```python
from build123d import *

# Parameters (mm, degrees)
F0_W     = 139.7
F0_H     = 241.3
F0_R     = 7.14375
F1_DEPTH = 12.7
F3_W     = 101.6
F3_H     = 203.2
F4_DEPTH = 12.7
F5_W     = 139.7
F5_H     = 12.7
F6_DEPTH = 244.602
F9_DEPTH = 215.901


with BuildPart() as f1:
    # F0 (on Top) → F1 (new body)
    with BuildSketch(Plane.XY):
        Rectangle(F0_W, F0_H)
        with Locations((-50.8, -63.5)):
            Circle(F0_R, mode=Mode.SUBTRACT)
        with Locations((50.8, -63.5)):
            Circle(F0_R, mode=Mode.SUBTRACT)
        with Locations((-50.8, 63.5)):
            Circle(F0_R, mode=Mode.SUBTRACT)
        with Locations((50.8, 63.5)):
            Circle(F0_R, mode=Mode.SUBTRACT)
    extrude(amount=F1_DEPTH)


with BuildPart() as f4:
    # F3 (on offset) → F4 (new body)
    with BuildSketch(Plane.XY.offset(270.002)):
        with Locations((-19.05, 0)):
            Rectangle(F3_W, F3_H)
        with BuildLine():
            ThreePointArc((-57.15, -65.913), (-62.738, -60.325), (-57.15, -54.737))
            Line((-57.15, -54.737), (19.05, -54.737))
            ThreePointArc((19.05, -54.737), (24.638, -60.325), (19.05, -65.913))
            Line((19.05, -65.913), (-57.15, -65.913))
        make_face(mode=Mode.SUBTRACT)
        with BuildLine():
            Line((19.05, 54.737), (-57.15, 54.737))
            ThreePointArc((-57.15, 54.737), (-62.738, 60.325), (-57.15, 65.913))
            Line((-57.15, 65.913), (19.05, 65.913))
            ThreePointArc((19.05, 65.913), (24.638, 60.325), (19.05, 54.737))
        make_face(mode=Mode.SUBTRACT)
    extrude(amount=-F4_DEPTH)


with BuildPart() as f6:
    # F5 (on face) → F6 (new body, through all)
    with BuildSketch(Plane.XY.offset(12.7)):
        with Locations((0, 88.9)):
            Rectangle(F5_W, F5_H)
    extrude(amount=F6_DEPTH)


with BuildPart() as f6b:
    # F5 (on face) → F6, piece 2 (new body, through all)
    with BuildSketch(Plane.XY.offset(12.7)):
        with Locations((0, -88.9)):
            Rectangle(F5_W, F5_H)
    extrude(amount=F6_DEPTH)


with BuildPart() as f1_1:
    add(f1.part)

    # F7: union F6b, F6, F4
    add(f6b.part)
    add(f6.part)
    add(f4.part)

    # F8 (on face) → F9 (cut, through all)
    with BuildSketch(Plane.XZ.offset(95.25)):
        Polygon((69.85, 257.302), (31.75, 257.302), (69.85, 12.7), align=None)
    extrude(amount=-F9_DEPTH, mode=Mode.SUBTRACT)


solid = f1_1.part
```
For this review, take the finished solid that the model builds, in its own axes (mm). A direction names the side the tool comes from. Round coordinates to 2 decimals unless told otherwise and drop trailing zeros. Write each loop counter-clockwise with the first axis right and the second up, starting at its lowest first coordinate (ties: lowest second). Pieces come first, ordered by that corner, then holes. Notation, with made-up numbers: (55.5, 21) - (59.5, 21) arc R34 ccw to (59.5, 57) - close; hole circle Ø7 at (73.5, 87.25). An arc over 180 degrees is marked (long way). Use CSV: the item, a comma, the result in double quotes.
1) For faces 4 (the flat face through (31.75, -1, 264)), 5 (the flat face through (-17, 82.55, 133)), 6 (the flat face through (-20, -54.737, 264)), list the 3-axis set-ups (+Z, -Z, +X, -X, +Y, -Y) from which the entire face can be reached by the end or side of a thin tool; tool diameter is ignored.
Conclusion:
face 4,"+Z, +X, +Y, -Y"
face 5,"+X, -X"
face 6,"+Z"
2) Add section D-D on x = -24.5. Write out the cut boundary in (y, z).
Conclusion:
outline,"(-120.65, 0) - (120.65, 0) - (120.65, 12.7) - (95.25, 12.7) - (95.25, 257.3) - (101.6, 257.3) - (101.6, 270) - (65.91, 270) - (65.91, 257.3) - (82.55, 257.3) - (82.55, 12.7) - (-82.55, 12.7) - (-82.55, 257.3) - (-65.91, 257.3) - (-65.91, 270) - (-101.6, 270) - (-101.6, 257.3) - (-95.25, 257.3) - (-95.25, 12.7) - (-120.65, 12.7) - close; (-54.74, 257.3) - (54.74, 257.3) - (54.74, 270) - (-54.74, 270) - close"
3) Add section B-B on x = -50.8. Count the separate pieces of the cut face and the enclosed holes in it, and give its area (3 significant figures).
Conclusion:
separate pieces,"4"
enclosed holes,"0"
area,"11,200 mm^2"
4) The part is to be moulded in two halves that separate along X. For faces 1 (the flat face through (69.85, -2, 6)), 2 (the flat face through (-17, 95.25, 133)), 3 (the flat face through (-19, -65.913, 264)), say which applies: pulls with the +X half, pulls with the -X half, needs draft (parallel to the pull), parting line crosses it, or undercut.
Conclusion:
face 1,"pulls with the +X half"
face 2,"needs draft"
face 3,"undercut"
5) Add section A-A on y = -38. Write out the cut boundary in (x, z).
Conclusion:
outline,"(-69.85, 0) - (69.85, 0) - (69.85, 12.7) - (-69.85, 12.7) - close; (-69.85, 257.3) - (31.75, 257.3) - (31.75, 270) - (-69.85, 270) - close"
6) Wall thickness on line 1 along Y through (x, z) = (-50, 6); line 2 along X through (y, z) = (63, 5); line 3 along Z through (x, y) = (8.5, -31): over which ranges is each line inside the solid? List them lowest first. Write a range as from..to.
Conclusion:
line 1,"y = -120.65..-70.6, -56.4..56.4, 70.6..120.65"
line 2,"x = -69.85..-57.93, -43.67..43.67, 57.93..69.85"
line 3,"z = 0..12.7, 257.3..270"
7) Clearance check with flat-ended pins moving along their axes: pin 1 Ø10 at (x, y) = (38, 73.5) entering from +Z; pin 2 Ø10 at (x, z) = (-1.5, 263) entering from +Y; pin 3 Ø6.5 at (x, z) = (-1, 266) entering from -Y. State where each tip first meets the part, or that it passes through.
Conclusion:
pin 1,"stops at z = 12.7"
pin 2,"stops at y = 101.6"
pin 3,"stops at y = -101.6"
8) Add section C-C on z = 198. Write out the cut boundary in (x, y), and give its area (3 significant figures).
Conclusion:
outline,"(-69.85, -95.25) - (40.99, -95.25) - (40.99, -82.55) - (-69.85, -82.55) - close; (-69.85, 82.55) - (40.99, 82.55) - (40.99, 95.25) - (-69.85, 95.25) - close"
area,"2,820 mm^2"
